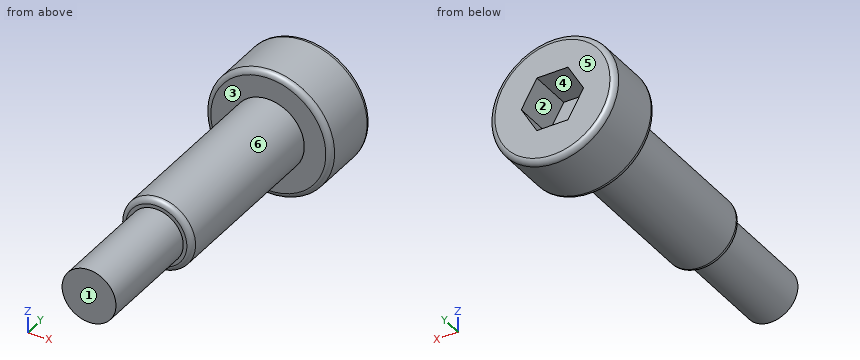
from build123d import *

# Parameters (mm, degrees)
FILLET_1_R          = 0.3
CUT_EXTRUDE_1_DEPTH = 2.4


with BuildPart() as part:
    # 草图1 → 旋转1 (revolve)
    with BuildSketch(Plane.XY):
        Polygon((0, 0), (-1.5, 0), (-1.5, 6), (-2, 6), (-2, 16), (-3.5, 16), (-3.5, 19.5), (0, 19.5), align=None)
    revolve(axis=Axis((0, 19.5, 0), (0, -1, 0)))

    # 圆角1
    fillet_1_edges = [part.edges().sort_by_distance(p)[0] for p in [
        (3.5, 19.5, 0),
        (3.5, 16, 0),
        (2, 6, 0),
    ]]
    fillet(fillet_1_edges, radius=FILLET_1_R)

    # 草图2 → 切除-拉伸1 (cut)
    with BuildSketch(Plane(origin=(0, 19.5, 0), x_dir=(1, 0, 0), z_dir=(0, 1, 0))):
        Polygon((0.866025404, -1.5), (1.732050808, 0), (0.866025404, 1.5), (-0.866025404, 1.5), (-1.732050808, 0), (-0.866025404, -1.5), align=None)
    extrude(amount=-CUT_EXTRUDE_1_DEPTH, mode=Mode.SUBTRACT)


solid = part.part
CAD build for the part. Positions are in the model's coordinates, mm. Face numbers are marked on the shaded views. A direction names the side the tool comes from. Round coordinates to 2 decimals unless told otherwise and drop trailing zeros. Write each loop counter-clockwise with the first axis right and the second up, starting at its lowest first coordinate (ties: lowest second). Pieces come first, ordered by that corner, then holes. Notation, with made-up numbers: M 64.5,-17.5 L 68.5,-17.5 A13 cw 68.5,4.5 Z; hole C 24.25,22.25 d8. An arc over 180 degrees is marked long. Use a Markdown table: item, result. Add a question column.
1. Flat gauge pins, fed straight in: P1, Ø4, axis at x = -2.5, y = 2, coming from the -Z side; P2, Ø4, axis at y = 10.5, z = 0.5, coming from the -X side. Where does each tip first touch, or does it go through?
2. Drill centre lines: probe 1 along Y at (x, z) = (-3, 0.5); probe 2 along X at (y, z) = (18.25, -1.25); probe 3 along Y at (x, z) = (1.5, -0.5). Where is each one in solid material? Low to high.
3. 3-axis set-ups, long thin cutter, end or side, ignore diameter. For the marked faces 1, 2 and 3: which of +Z, -Z, +X, -X, +Y, -Y reach the whole face in a straight line?
4. Slice it at B-B on x = 0. Give the cut face in (y, z), then the cut area to 3 significant figures.
5. Slice it at D-D on y = 2.75. Give the cut face in (x, z).
6. Slice it at C-C on y = 11.75. Give the cut face in (x, z).
7. Slice it at A-A on y = 17.5. Give the cut face in (x, z).
8. Pull direction X, two halves, no side cores. Call the marked faces 4, 5 and 6: released by +X, released by -X, zero draft, split by the parting line, or undercut.
Reply:
| question | item | result |
|---|---|---|
| 1 | P1 | stops at z = -1.41 |
| 1 | P2 | stops at x = -2 |
| 2 | probe 1 | y = 16 to 19.5 |
| 2 | probe 2 | x = -3.27 to -1.01, 1.01 to 3.27 |
| 2 | probe 3 | y = 6 to 19.5 |
| 3 | face 1 | +Z, -Z, +X, -X, -Y |
| 3 | face 2 | +Y |
| 3 | face 3 | -Y |
| 4 | outline | M 0,-1.5 L 6,-1.5 L 6,-1.7 A0.3 ccw 6.3,-2 L 16,-2 L 16,-3.2 A0.3 ccw 16.3,-3.5 L 19.2,-3.5 A0.3 ccw 19.5,-3.2 L 19.5,-1.5 L 17.1,-1.5 L 17.1,1.5 L 19.5,1.5 L 19.5,3.2 A0.3 ccw 19.2,3.5 L 16.3,3.5 A0.3 ccw 16,3.2 L 16,2 L 6.3,2 A0.3 ccw 6,1.7 L 6,1.5 L 0,1.5 Z |
| 4 | area | 75.2 mm^2 |
| 5 | outline | C 0,0 d3 |
| 6 | outline | C 0,0 d4 |
| 7 | outline | C 0,0 d7; hole M -1.73,0 L -0.87,-1.5 L 0.87,-1.5 L 1.73,0 L 0.87,1.5 L -0.87,1.5 Z |
| 8 | face 4 | undercut |
| 8 | face 5 | zero draft |
| 8 | face 6 | split by the parting line |
